```python
from build123d import *

# Parameters (mm, degrees)
ESQUISSE1_W        = 20
ESQUISSE1_H        = 5
BOSS_EXTRU_1_DEPTH = 10
CONG_1_R           = 5


with BuildPart() as part:
    # Esquisse1 → Boss.-Extru.1 (new body)
    with BuildSketch(Plane.XY):
        with Locations((10, 2.5)):
            Rectangle(ESQUISSE1_W, ESQUISSE1_H)
    extrude(amount=BOSS_EXTRU_1_DEPTH)

    # Congé1
    cong_1_edges = [part.edges().sort_by_distance(p)[0] for p in [
        (20, 5, 5),
    ]]
    fillet(cong_1_edges, radius=CONG_1_R - 0.0001)  # a hair under: the kernel refuses the full size


solid = part.part
```
Model file for the job. Use its own axes, mm. Give positions to 0.01 mm unless a question says otherwise; leave off trailing zeros. Write each loop counter-clockwise with the first axis right and the second up, starting at its lowest first coordinate (ties: lowest second). Pieces come first, ordered by that corner, then holes. Notation, with made-up numbers: (-39, -5.75) - (2, -5.75) arc R27 ccw to (2, 24.25) - close; hole circle Ø4 at (80, -19.5). An arc over 180 degrees is marked (long way). One line per question, with ' | ' between items. Start each with the question number.
(1) Pin check, flat tip, straight feed: P1, Ø1, axis at x = 11.5, z = 9, coming from the -Y side. Stop position of the tip, or through.
(2) Slice it at B-B on y = 2.7. Write the cut outline in (x, z), plus the area to 3 significant figures.
(3) Slice it at C-C on x = 18. Write the cut outline in (y, z), plus the area to 3 significant figures.
(4) Wall check: line 1 along X through (y, z) = (1.75, 9.25); line 2 along Y through (x, z) = (19, 7); line 3 along X through (y, z) = (0.7, 3). Give the ranges that are in metal, low to high. Write a range as from..to.
Results below:
1) P1: y = 0
2) outline: (0, 0) - (19.21, 0) - (19.21, 10) - (0, 10) - close | area: 192 mm^2
3) outline: (0, 0) - (4, 0) - (4, 10) - (0, 10) - close | area: 40.0 mm^2
4) line 1: 0..19.68 | line 2: 0..3 | line 3: 0..19.95
